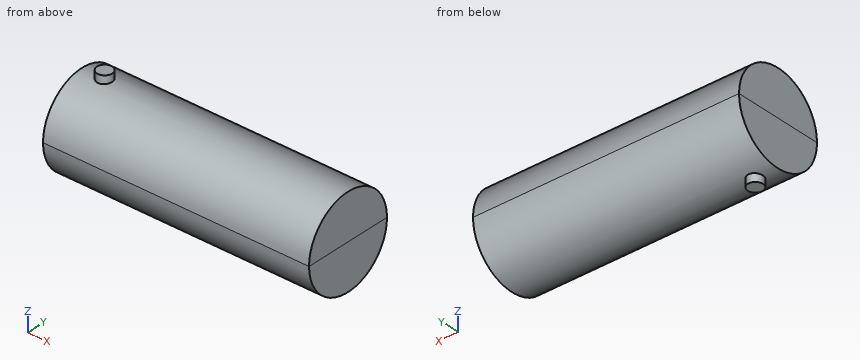
from build123d import *
from build123d import SkipClean  # not in build123d's __all__

# Parameters (mm, degrees)
F1_DEPTH = 8.8
F2_R     = 0.25
F3_DEPTH = 1.75


with BuildPart() as f1:
    # F0 (on Right) → F1 (new body)
    with BuildSketch(Plane.YZ):
        with BuildLine():
            Line((-1.5, 0), (1.5, 0))
            ThreePointArc((1.5, 0), (0, 1.5), (-1.5, 0))
        make_face()
    extrude(amount=F1_DEPTH)

    # F2 (on face) → F3 (join, symmetric)
    with BuildSketch(Plane(origin=(0, 0, 0), x_dir=(1, 0, 0), z_dir=(0, 0, -1))):
        with Locations((0.75, 0)):
            Circle(F2_R)
    extrude(amount=F3_DEPTH, both=True)

    # F4: F1 across plane


with BuildPart() as f1_1:
    add(f1.part, clean=False)
    with SkipClean():  # cleaning this boolean's faces spoils the solid; the shape is the same uncleaned
        add(f1.part.mirror(Plane.XY), clean=False)


solid = f1_1.part
Part model, mm, in its own coordinate system. Coordinates: 2 decimals unless noted, no trailing zeros. Order: outer loops, then holes, each group sorted by start corner. A loop starts at its lowest first (then second) coordinate and runs counter-clockwise, first axis right, second up.
(1) Pin check, flat tips, straight feed: pin 1 Ø1 at (x, y) = (4.5, 1) entering from +Z; pin 2 Ø1 at (x, y) = (2, -0.5) entering from +Z; pin 3 Ø1 at (x, y) = (3, 0) entering from -Z. Stop position of each tip, or through.
Check sheet entries:
pin 1: stops at z = 1.41
pin 2: stops at z = 1.5
pin 3: stops at z = -1.5
(2) Probe L1, parallel to Y at x = 3.25, z = 0.25; L2, parallel to Z at x = 8.25, y = -0.6; L3, parallel to Y at x = 4, z = -1.3. List the from-to ranges inside material, lowest first.
Check sheet entries:
L1: y = -1.48 to 1.48
L2: z = -1.37 to 1.37
L3: y = -0.75 to 0.75
(3) Slice it at A-A, the plane x = 0.75. Write the cut outline in (y, z), and give its area (3 significant figures).
Check sheet entries:
outline: (-0.25, -1.75) - (0.25, -1.75) - (0.25, -1.48) arc R1.5 ccw to (0.25, 1.48) - (0.25, 1.75) - (-0.25, 1.75) - (-0.25, 1.48) arc R1.5 ccw to (-0.25, -1.48) - close
area: 7.33 mm2
(4) Slice it at C-C, the plane z = 1. Write the cut outline in (x, y), and give its area (3 significant figures).
Check sheet entries:
outline: (0, -1.12) - (8.8, -1.12) - (8.8, 1.12) - (0, 1.12) - close
area: 19.7 mm2
(5) Slice it at D-D, the plane z = 0.3. Write the cut outline in (x, y), and give its area (3 significant figures).
Check sheet entries:
outline: (0, -1.47) - (8.8, -1.47) - (8.8, 1.47) - (0, 1.47) - close
area: 25.9 mm2
(6) Slice it at B-B, the plane y = 0. Write the cut outline in (x, z), and give its area (4 significant figures).
Check sheet entries:
outline: (0, -1.5) - (0.5, -1.5) - (0.5, -1.75) - (1, -1.75) - (1, -1.5) - (8.8, -1.5) - (8.8, 1.5) - (1, 1.5) - (1, 1.75) - (0.5, 1.75) - (0.5, 1.5) - (0, 1.5) - close
area: 26.65 mm2
